Geometry check sheet. Reference: the model listing, model coordinates, mm. A direction names the side the tool comes from. Round coordinates to 2 decimals unless told otherwise and drop trailing zeros. Order: outer loops, then holes, each group sorted by start corner. A loop starts at its lowest first (then second) coordinate and runs counter-clockwise, first axis right, second up.
(1) Cross-section at D-D on y = -14. Enter the section's corners in (x, z).
(2) Cross-section at B-B on y = 0. Enter the section's corners in (x, z).
(3) Gauge pin test, flat ends, axial feed: P1, Ø8, axis at y = 2.5, z = -13, coming from the -X side; P2, Ø2, axis at x = 12.5, y = 4, coming from the -Z side; P3, Ø10, axis at x = 11.5, z = -11.5, coming from the +Y side; P4, Ø6, axis at x = -4, z = -4, coming from the -Y side. Record the tip position at first contact, or that the pin passes through.
(4) Draft check along Y on faces 4 (the face through (0, -4, 2.362)), 5 (the face through (14.3, -4.26, 0.03)), 6 (the face through (-10.43, -17.81, 0.03)). Enter one of: pulls with the +Y half, pulls with the -Y half, needs draft (parallel to the pull), parting line crosses it, or undercut.
(5) Thickness scan on L1, parallel to Y at x = 0, z = -9.75; L2, parallel to Z at x = 8, y = -6; L3, parallel to Y at x = 0, z = 0.5. Record the ranges inside material, lowest first.
(6) Cross-section at A-A on z = 0.5. Enter the section's corners in (x, y) (1 decimal).
(7) Cross-section at C-C on x = 0. Enter the section's corners in (y, z), and give its area (3 significant figures).
(8) Set-up check for faces 1 (the face through (10.43, 17.81, 0.03)), 2 (the face through (0, -9, -2.362)), 3 (the face through (1.1, -15.06, 0.03)): record each of +Z, -Z, +X, -X, +Y, -Y from which the full face is reachable in a straight line by a thin tool's end or side.
from build123d import *

# Parameters (mm, degrees)
SKETCH1_R           = 20.6375
BOSS_EXTRUDE1_DEPTH = 2.3622
CUT_EXTRUDE1_DEPTH  = 30.565736383
SKETCH4_R           = 8.5725
BOSS_EXTRUDE2_DEPTH = 12.7
CIRPATTERN1_COUNT   = 6
CUT_EXTRUDE2_DEPTH  = 34.954416084
CHAMFER1_SIZE       = 0.7874


with BuildPart() as part:
    # Sketch1 → Boss-Extrude1 (new, symmetric)
    with BuildSketch(Plane.XY):
        Circle(SKETCH1_R)
    extrude(amount=BOSS_EXTRUDE1_DEPTH, both=True)

    # Sketch2 → Cut-Extrude1 (cut, through all)
    with BuildSketch(Plane.XY.offset(2.3622)):
        with BuildLine():
            Line((-2.397761805, 8.89), (-3.877589744, 8.351386678))
            ThreePointArc((-3.877589744, 8.351386678), (-3.446754472, 14.597661325), (-1.5875, 20.576351717))
            ThreePointArc((-1.5875, 20.576351717), (0, 20.6375), (1.5875, 20.576351717))
            ThreePointArc((1.5875, 20.576351717), (-1.12604651, 14.979021398), (-2.397761805, 8.89))
        make_face()
    cut_extrude1 = extrude(amount=-CUT_EXTRUDE1_DEPTH, mode=Mode.SUBTRACT)

    # Sketch4 → Boss-Extrude2 (add)
    with BuildSketch(Plane(origin=(0, 0, -2.3622), x_dir=(-1, 0, 0), z_dir=(0, 0, -1))):
        with Locations(Location((0, 0, 0), (0, 0, 180))):
            Circle(SKETCH4_R)
    extrude(amount=BOSS_EXTRUDE2_DEPTH)

    # CirPattern1: Cut-Extrude1 ×6 about axis
    cirpattern1_axis = Axis((0, 0, 0), (0, 0, 1))
    for i in range(1, CIRPATTERN1_COUNT):
        add(cut_extrude1.rotate(cirpattern1_axis, i * 360 / CIRPATTERN1_COUNT), mode=Mode.SUBTRACT)

    # Sketch3 → Cut-Extrude2 (cut, through all)
    with BuildSketch(Plane.XY.offset(2.3622)):
        with BuildLine():
            Line((-1.658312395, 2.5), (1.658312395, 2.5))
            ThreePointArc((1.658312395, 2.5), (0, -3), (-1.658312395, 2.5))
        make_face()
    extrude(amount=-CUT_EXTRUDE2_DEPTH, mode=Mode.SUBTRACT)

    # Chamfer1
    chamfer1_edges = [part.edges().sort_by_distance(p)[0] for p in [
        (-8.5725, 0, -15.0622),
    ]]
    chamfer(chamfer1_edges, length=CHAMFER1_SIZE)


solid = part.part
Found:
1. outline: (-15.16, -2.36) - (1.44, -2.36) - (1.44, 2.36) - (-15.16, 2.36) - close; (3.55, -2.36) - (15.16, -2.36) - (15.16, 2.36) - (3.55, 2.36) - close
2. outline: (-20.64, -2.36) - (-8.57, -2.36) - (-8.57, -14.27) - (-7.79, -15.06) - (-3, -15.06) - (-3, 2.36) - (-20.64, 2.36) - close; (3, -15.06) - (7.79, -15.06) - (8.57, -14.27) - (8.57, -2.36) - (20.64, -2.36) - (20.64, 2.36) - (3, 2.36) - close
3. P1: stops at x = -8.57
3. P2: stops at z = -2.36
3. P3: stops at y = 5.59
3. P4: stops at y = -20.58
4. face 4: needs draft
4. face 5: undercut
4. face 6: pulls with the -Y half
5. L1: y = -8.57 to -3, 2.5 to 8.57
5. L2: z = -2.36 to 2.36
5. L3: y = -17.74 to -3, 2.5 to 17.74
6. outline: (-18.6, -8.9) arc R25.4 ccw to (-6.5, -6.5) - (-5.3, -7.5) arc R27 cw to (-17, -11.7) arc R20.6 ccw to (-1.6, -20.6) arc R25.4 ccw to (2.4, -8.9) - (3.9, -8.4) arc R27 cw to (1.6, -20.6) arc R20.6 ccw to (17, -11.7) arc R25.4 ccw to (8.9, -2.4) - (9.2, -0.8) arc R27 cw to (18.6, -8.9) arc R20.6 ccw to (18.6, 8.9) arc R25.4 ccw to (6.5, 6.5) - (5.3, 7.5) arc R27 cw to (17, 11.7) arc R20.6 ccw to (1.6, 20.6) arc R25.4 ccw to (-2.4, 8.9) - (-3.9, 8.4) arc R27 cw to (-1.6, 20.6) arc R20.6 ccw to (-17, 11.7) arc R25.4 ccw to (-8.9, 2.4) - (-9.2, 0.8) arc R27 cw to (-18.6, 8.9) arc R20.6 ccw to start; hole (-1.7, 2.5) arc R3 ccw (long way) to (1.7, 2.5) - close
7. outline: (-17.74, -2.36) - (-8.57, -2.36) - (-8.57, -14.27) - (-7.79, -15.06) - (-3, -15.06) - (-3, 2.36) - (-17.74, 2.36) - close; (2.5, -15.06) - (7.79, -15.06) - (8.57, -14.27) - (8.57, -2.36) - (17.74, -2.36) - (17.74, 2.36) - (2.5, 2.36) - close
7. area: 289 mm2
8. face 1: +Z, -Z, +X, +Y
8. face 2: -Z
8. face 3: +Z, -Z
